```python
from build123d import *

# Parameters (mm, degrees)
EXTRUDE3_DEPTH     = 17.78
SKETCH8_R          = 1.5875
CUT_EXTRUDE4_DEPTH = 17.78
SKETCH9_W          = 17.78
SKETCH9_H          = 260.35
SKETCH9_H_2        = 189.179603175
SKETCH9_W_2        = 146.050000002
SKETCH9_H_3        = 17.78
CUT_EXTRUDE5_DEPTH = 5.08


with BuildPart() as part:
    # Sketch7 → Extrude3 (new body)
    with BuildSketch(Plane.XY):
        Polygon((157.1625, -6013.45), (857.25, -6013.45), (857.25, -5826.125), (157.1625, -5753.1), align=None)
    extrude(amount=-EXTRUDE3_DEPTH)

    # Sketch8 → Cut-Extrude4 (cut)
    with BuildSketch(Plane.XY):
        with Locations((166.0525, -5970.212883599)):
            Circle(SKETCH8_R)
        with Locations((166.0525, -5883.738650795)):
            Circle(SKETCH8_R)
        with Locations((166.0525, -5797.264417991)):
            Circle(SKETCH8_R)
        with Locations((848.36, -5982.074616401)):
            Circle(SKETCH8_R)
        with Locations((848.36, -5919.323849205)):
            Circle(SKETCH8_R)
        with Locations((848.36, -5856.573082009)):
            Circle(SKETCH8_R)
        with Locations((471.4875, -5910.834)):
            Circle(SKETCH8_R)
        with Locations((522.2875, -5910.834)):
            Circle(SKETCH8_R)
        with Locations((573.0875, -5910.834)):
            Circle(SKETCH8_R)
    extrude(amount=-CUT_EXTRUDE4_DEPTH, mode=Mode.SUBTRACT)

    # Sketch9 → Cut-Extrude5 (cut)
    with BuildSketch(Plane.XY):
        with Locations((166.0525, -5883.275)):
            Rectangle(SKETCH9_W, SKETCH9_H)
        with Locations((848.36, -5918.860198413)):
            Rectangle(SKETCH9_W, SKETCH9_H_2)
        with Locations((522.2875, -5910.834)):
            Rectangle(SKETCH9_W_2, SKETCH9_H_3)
    extrude(amount=-CUT_EXTRUDE5_DEPTH, mode=Mode.SUBTRACT)


solid = part.part
```
Could you check a few things on this model? Use its own coordinates, in mm. A direction names the side the tool comes from. Coordinates: 2 decimals unless noted, no trailing zeros. Loops run counter-clockwise (first coordinate to the right, second up) from the corner with the lowest first, then second, coordinate; pieces in that order, holes last.
1) Imagine slicing it at B-B (x = 809). List the corners of the cut face in (y, z) for me, and give its area (3 significant figures).
Reported:
outline: (-6013.45, -17.78) - (-5821.09, -17.78) - (-5821.09, 0) - (-6013.45, 0) - close
area: 3,420 mm2
2) Which directions (+Z, -Z, +X, -X, +Y, -Y) give clear straight access to the entire face, cutting with the end or side of a thin tool? Please do faces 1 (the face through (502, -6013.45, -9)), 2 (the face through (848.2, -5917.5, -5.08)), 3 (the face through (166, -5881, -5.08)).
Reported:
face 1: +Z, -Z, +X, -X, -Y
face 2: +Z, +X, +Y, -Y
face 3: +Z, -X, +Y, -Y
3) Thinking about a two-plate mould opening in Y: for faces 4 (the face through (521, -5909, -5.08)), 5 (the face through (857.25, -5921, -11)), 6 (the face through (512.107, -5790.124, -8.766)), which applies, released by +Y, released by -Y, zero draft, split by the parting line, or undercut?
Reported:
face 4: undercut
face 5: zero draft
face 6: released by +Y
4) Imagine slicing it at A-A (z = -13.5). State how many separate pieces and enclosed holes the cut face has, and give its area (3 significant figures).
Reported:
separate pieces: 1
enclosed holes: 9
area: 157,000 mm2
5) Please list where these lines run through material, in increasing order: line 1 along Y through (x, z) = (848.36, -13); line 2 along X through (y, z) = (-5918, -5); line 3 along X through (y, z) = (-5983, -10.5).
Reported:
line 1: y = -6013.45 to -5983.66, -5980.49 to -5920.91, -5917.74 to -5858.16, -5854.99 to -5825.2
line 2: x = 174.94 to 449.26, 595.31 to 839.47
line 3: x = 157.16 to 847.07, 849.65 to 857.25
6) Imagine slicing it at C-C (x = 224.5). List the corners of the cut face in (y, z) for me, and give its area (3 significant figures).
Reported:
outline: (-6013.45, -17.78) - (-5760.12, -17.78) - (-5760.12, 0) - (-6013.45, 0) - close
area: 4,500 mm2
7) Will these pins go through, and if not, where does the flat tip stop? pin 1 Ø1.5 at (x, z) = (344, -8.5) entering from +Y; pin 2 Ø2.5 at (y, z) = (-5915, -2) entering from +X; pin 3 Ø5.5 at (x, z) = (512.5, -3) entering from +Y.
Reported:
pin 1: stops at y = -5772.51
pin 2: stops at x = 839.47
pin 3: stops at y = -5789.88
